Source: CAD feature listing. Evaluate the final solid. Frame: model axes, mm. Face numbers are marked on the shaded views. A direction names the side the tool comes from. Give positions to 0.01 mm unless a question says otherwise; leave off trailing zeros. Loops run counter-clockwise (first coordinate to the right, second up) from the corner with the lowest first, then second, coordinate; pieces in that order, holes last. Notation, with made-up numbers: M -35.5,-14.75 L 4.5,-14.75 A22 ccw 4.5,2.25 Z; hole C -26,73 d9. An arc over 180 degrees is marked long. Answer in a Markdown table with one row per item.
```python
from build123d import *

# Parameters (mm, degrees)
F1_DEPTH = 7.5
F2_W     = 28.4275773028
F2_H     = 3.6
F3_DEPTH = 10.201
F5_DEPTH = 7.5


with BuildPart() as f1:
    # F0 (on Top) → F1 (new body)
    with BuildSketch(Plane.XY):
        with BuildLine():
            ThreePointArc((0, 10.2), (-5.1, 5.1), (0, 0))
            Line((0, 0), (0, 2.6))
            ThreePointArc((0, 2.6), (-2.5, 5.1), (0, 7.6))
            Line((0, 7.6), (0, 10.2))
        make_face()
        with BuildLine():
            Line((-29.2, 0), (0, 0))
            ThreePointArc((0, 0), (-5.1, 5.1), (0, 10.2))
            Line((0, 10.2), (-29.2, 10.2))
            ThreePointArc((-29.2, 10.2), (-25.5937554159, 8.7062445841), (-24.1, 5.1))
            ThreePointArc((-24.1, 5.1), (-25.5937554159, 1.4937554159), (-29.2, 0))
        make_face()
        with BuildLine():
            Line((0, 2.6), (0, 0))
            ThreePointArc((0, 0), (3.6062445841, 1.4937554159), (5.1, 5.1))
            ThreePointArc((5.1, 5.1), (3.6062445841, 8.7062445841), (0, 10.2))
            Line((0, 10.2), (0, 7.6))
            ThreePointArc((0, 7.6), (1.767766953, 6.867766953), (2.5, 5.1))
            ThreePointArc((2.5, 5.1), (1.767766953, 3.332233047), (0, 2.6))
        make_face()
        with BuildLine():
            ThreePointArc((-29.2, 10.2), (-34.3, 5.1), (-29.2, 0))
            Line((-29.2, 0), (-29.2, 2.6))
            ThreePointArc((-29.2, 2.6), (-31.7, 5.1), (-29.2, 7.6))
            Line((-29.2, 7.6), (-29.2, 10.2))
        make_face()
        with BuildLine():
            Line((-29.2, 2.6), (-29.2, 0))
            ThreePointArc((-29.2, 0), (-25.5937554159, 1.4937554159), (-24.1, 5.1))
            ThreePointArc((-24.1, 5.1), (-25.5937554159, 8.7062445841), (-29.2, 10.2))
            Line((-29.2, 10.2), (-29.2, 7.6))
            ThreePointArc((-29.2, 7.6), (-27.432233047, 6.867766953), (-26.7, 5.1))
            ThreePointArc((-26.7, 5.1), (-27.432233047, 3.332233047), (-29.2, 2.6))
        make_face()
    extrude(amount=F1_DEPTH)

    # F2 (on face) → F3 (cut, through all)
    with BuildSketch(Plane.XZ):
        with Locations((-2.2280919366, 3.75)):
            Rectangle(F2_W, F2_H)
    extrude(amount=-F3_DEPTH, mode=Mode.SUBTRACT)

    # F4 (on face) → F5 (join)
    with BuildSketch(Plane.XY.offset(7.5)):
        with BuildLine():
            ThreePointArc((-34.0871795985, 3.6420989157), (-33.913058879, 7.0486087353), (-31.6307227456, 9.5834793335))
            Line((-31.6307227456, 9.5834793335), (-46.8735157819, 15.4770560035))
            Line((-46.8735157819, 15.4770560035), (-49.1914411807, 9.4821128467))
            Line((-49.1914411807, 9.4821128467), (-34.0871795985, 3.6420989157))
        make_face()
    extrude(amount=-F5_DEPTH)


solid = f1.part
```
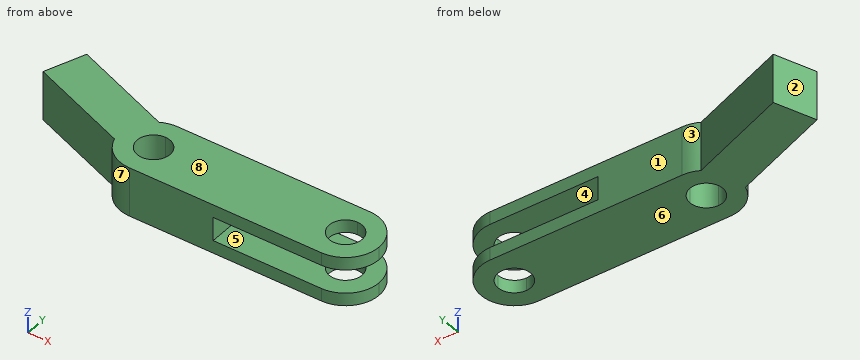
Q1. Section query B-B (y = 5.75). Output: boundary loops of the cut face in (x, z).
Values follow:
| item | result |
|---|---|
| outline | M -39.54,0 L -31.61,0 L -31.61,7.5 L -39.54,7.5 Z; M -26.79,0 L -2.41,0 L -2.41,1.95 L -16.44,1.95 L -16.44,5.55 L -2.41,5.55 L -2.41,7.5 L -26.79,7.5 Z; M 2.41,0 L 5.06,0 L 5.06,1.95 L 2.41,1.95 Z; M 2.41,5.55 L 5.06,5.55 L 5.06,7.5 L 2.41,7.5 Z |
Q2. Section query C-C (z = 6.25). Output: boundary loops of the cut face in (x, y), plus the area to 3 significant figures.
Values follow:
| item | result |
|---|---|
| outline | M -49.19,9.48 L -34.09,3.64 A5.1 ccw -29.2,0 L 0,0 A5.1 ccw 0,10.2 L -29.2,10.2 A5.1 ccw -31.63,9.58 L -46.87,15.48 Z; hole C -29.2,5.1 d5; hole C 0,5.1 d5 |
| area | 440 mm^2 |
Q3. Contact query for a flat-ended pin moving along its axis: pin 1 Ø3 at (x, z) = (-22.5, 6.5) entering from +Y. Output: stop coordinate, or through.
Values follow:
| item | result |
|---|---|
| pin 1 | y = 10.2 |
Q4. Ray query, probe 1 along Z at (x, y) = (-11.5, 5.5); probe 2 along Y at (x, z) = (-7, 6); probe 3 along X at (y, z) = (9.5, 2.75). Return the intervals inside material, ascending. Write a range as from..to.
Values follow:
| item | result |
|---|---|
| probe 1 | 0..1.95, 5.55..7.5 |
| probe 2 | 0..10.2 |
| probe 3 | -49.18..-16.44 |
Q5. Reachability of the marked faces 1, 2, 3 and 4 from +Z, -Z, +X, -X, +Y, -Y: full face, straight path, thin tool, end or side. Return the list, or none.
Values follow:
| item | result |
|---|---|
| face 1 | +Z, -Z, +X, +Y |
| face 2 | +Z, -Z, -X, +Y |
| face 3 | +Z, -Z, +Y |
| face 4 | +X, +Y, -Y |
Q6. Section query A-A (z = 4). Output: boundary loops of the cut face in (x, y).
Values follow:
| item | result |
|---|---|
| outline | M -49.19,9.48 L -34.09,3.64 A5.1 ccw -29.2,0 L -16.44,0 L -16.44,10.2 L -29.2,10.2 A5.1 ccw -31.63,9.58 L -46.87,15.48 Z; hole C -29.2,5.1 d5 |
Q7. Section query D-D (y = 2). Output: boundary loops of the cut face in (x, z).
Values follow:
| item | result |
|---|---|
| outline | M -33.25,0 L 4.05,0 L 4.05,1.95 L -16.44,1.95 L -16.44,5.55 L 4.05,5.55 L 4.05,7.5 L -33.25,7.5 Z |
Q8. Mould query, pull axis Z, two halves, no side actions, for the marked faces 5, 6, 7 and 8. Classes: +Z half, -Z half, draft (parallel to the pull), parting line (faces both ways), or undercut.
Values follow:
| item | result |
|---|---|
| face 5 | undercut |
| face 6 | -Z half |
| face 7 | draft |
| face 8 | +Z half |
